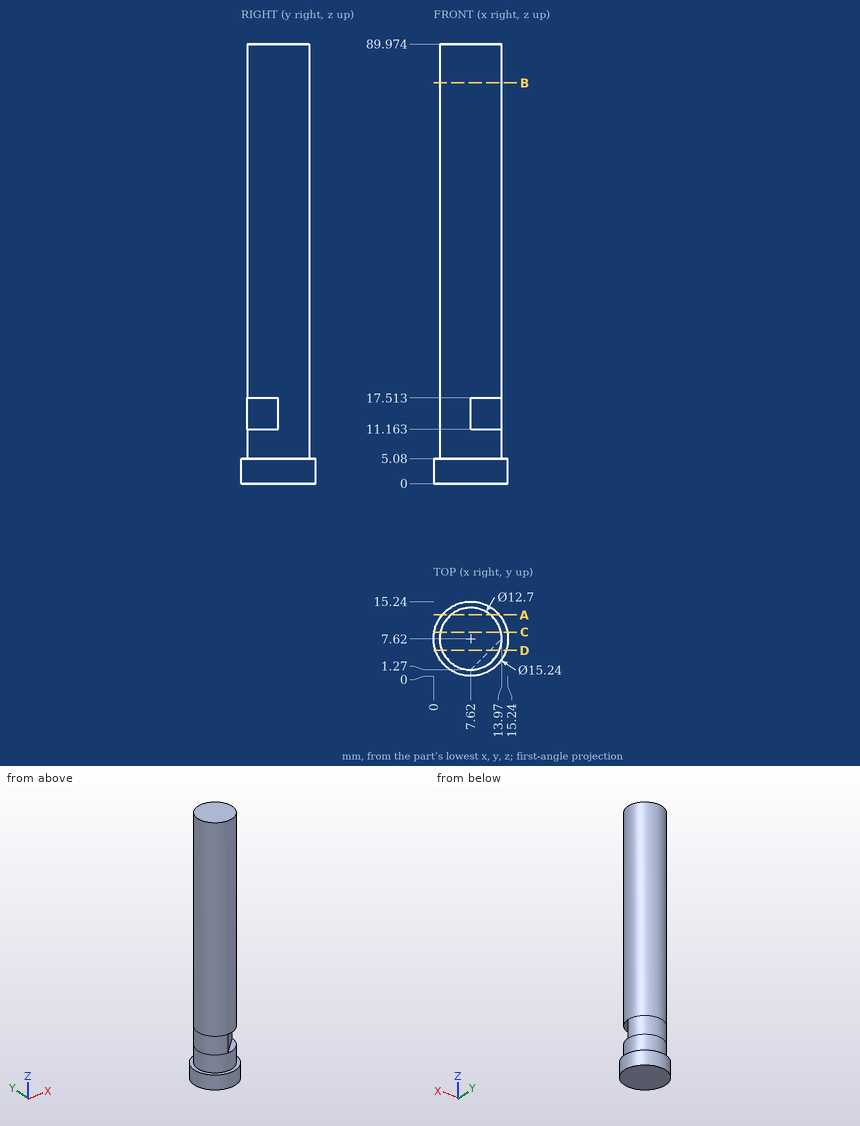
The drawing under review shows one solid part. Ordinate dimensions are in mm from its lowest x, y, z. Coordinates: 2 decimals unless noted, no trailing zeros. Order: outer loops, then holes, each group sorted by start corner. A loop starts at its lowest first (then second) coordinate and runs counter-clockwise, first axis right, second up. Notation, with made-up numbers: (-1.5, 14) -> (46.5, 14) arc R24 cw to (46.5, 32) -> close; hole circle Ø2 at (-27.75, 58). An arc over 180 degrees is marked (long way). Use CSV: the item, a comma, the result in double quotes. Start each with the question number.
Item 1: We need section C-C, the plane y = 9. Give the boundary of the cut face in (x, z) (1 decimal).
Item 2: We need section D-D, the plane y = 5.25. Give the boundary of the cut face in (x, z) (1 decimal), then the cut area to 3 significant figures.
Item 3: We need section A-A, the plane y = 12.5. Give the boundary of the cut face in (x, z) (1 decimal), then the cut area to 3 significant figures.
Item 4: Wall thickness on probe 1 along Z at (x, y) = (10.25, 3) (1 decimal); probe 2 along Y at (x, z) = (7.5, 81.5): over which ranges is each line inside the solid? List them lowest first.
Item 5: Insertion check: pin 1 (2 mm diameter, centred on x = 11, z = 68, fed in from +Y); pin 2 (4 mm diameter, centred on x = 3, z = 67.5, fed in from -Y) (1 decimal); pin 3 (1.5 mm diameter, centred on x = 10.5, y = 11, fed in from -Z); pin 4 (8 mm diameter, centred on y = 4, z = 50.5, fed in from -X). Each pin has a flat end and moves straight along its axis. Give the tip position at first contact, or say it passes through.
Item 6: We need section B-B, the plane z = 82. Give the boundary of the cut face in (x, y).
Derived:
1,outline,"(0.1, 0) -> (15.1, 0) -> (15.1, 5.1) -> (13.8, 5.1) -> (13.8, 90) -> (1.4, 90) -> (1.4, 5.1) -> (0.1, 5.1) -> close"
2,outline,"(0.4, 0) -> (14.9, 0) -> (14.9, 5.1) -> (13.5, 5.1) -> (13.5, 11.2) -> (11.6, 11.2) -> (11.6, 17.5) -> (13.5, 17.5) -> (13.5, 90) -> (1.7, 90) -> (1.7, 5.1) -> (0.4, 5.1) -> close"
2,area,"1,060 mm^2"
3,outline,"(1.8, 0) -> (13.5, 0) -> (13.5, 5.1) -> (11.7, 5.1) -> (11.7, 90) -> (3.6, 90) -> (3.6, 5.1) -> (1.8, 5.1) -> close"
3,area,"749 mm^2"
4,probe 1,"z = 0 to 11.2, 17.5 to 90"
4,probe 2,"y = 1.27 to 13.97"
5,pin 1,"stops at y = 13.51"
5,pin 2,"stops at y = 1.8"
5,pin 3,"stops at z = 0"
5,pin 4,"stops at x = 1.27"
6,outline,"circle Ø12.7 at (7.62, 7.62)"
